Input: dimensioned drawing with shaded views. Units: mm. Origin: part minimum x, y, z. Give positions to 0.01 mm unless a question says otherwise; leave off trailing zeros. Loops run counter-clockwise (first coordinate to the right, second up) from the corner with the lowest first, then second, coordinate; pieces in that order, holes last. Notation, with made-up numbers: (79.25, 57) -> (116.25, 57) arc R14 cw to (116.25, 68) -> close; hole circle Ø1 at (28, 26). An arc over 180 degrees is marked (long way). Answer in a Markdown table with one row per item. Add a question column.
1) Section query B-B (y = 1.5). Return the cut outline in (x, z).
2) Draft query along X for the marked faces 1, 2 and 3. Return one class per face: +X half, -X half, draft (parallel to the pull), parting line (faces both ways), or undercut.
3) Line query: line 1 (Y direction, x = 3.45, z = 1.65); line 2 (Z direction, x = 1.35, y = 6); line 3 (Y direction, x = 2.05, z = 2.2). Output: solid intervals per line, ascending. Write a range as from..to.
4) Section query A-A (y = 6.5). Return the cut outline in (x, z), plus the area to 3 significant figures.
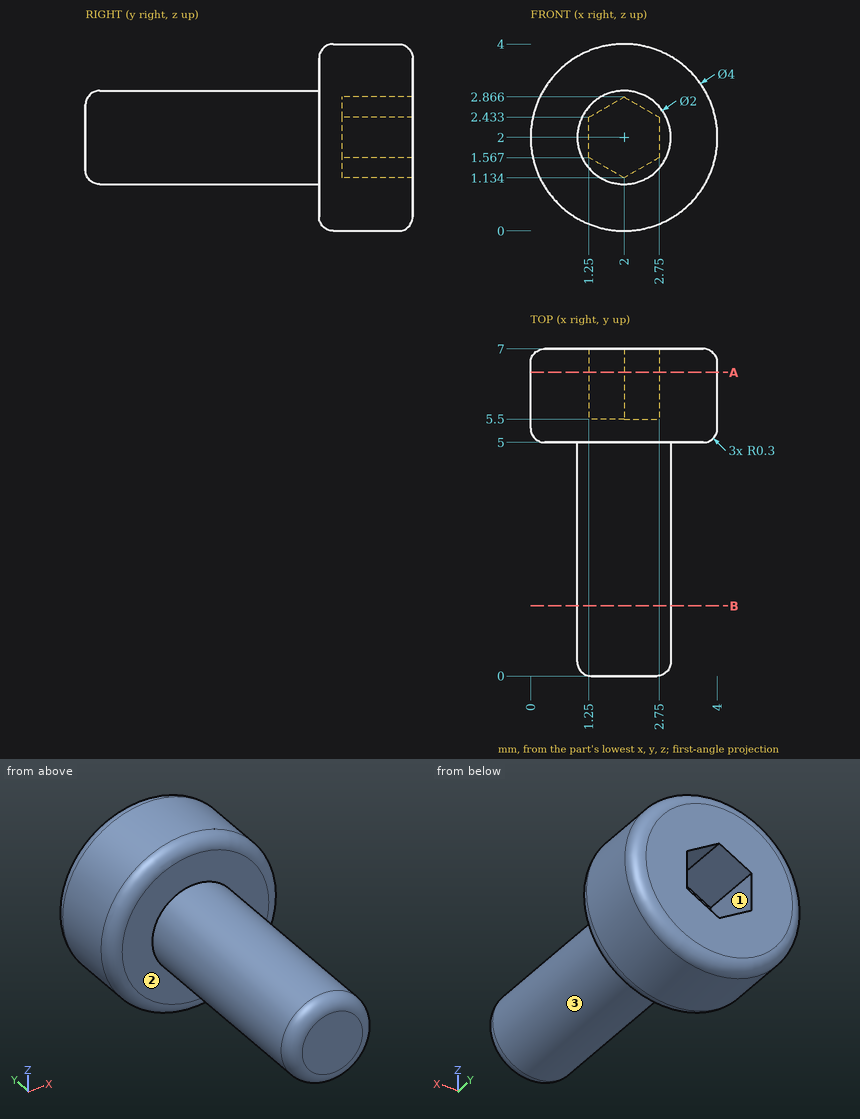
Evaluation:
| question | item | result |
|---|---|---|
| 1 | outline | circle Ø2 at (2, 2) |
| 2 | face 1 | undercut |
| 2 | face 2 | draft |
| 2 | face 3 | parting line |
| 3 | line 1 | 5..7 |
| 3 | line 2 | 0.11..1.51, 2.49..3.89 |
| 3 | line 3 | 0..5.5 |
| 4 | outline | circle Ø4 at (2, 2); hole (1.25, 1.57) -> (2, 1.13) -> (2.75, 1.57) -> (2.75, 2.43) -> (2, 2.87) -> (1.25, 2.43) -> close |
| 4 | area | 10.6 mm² |
